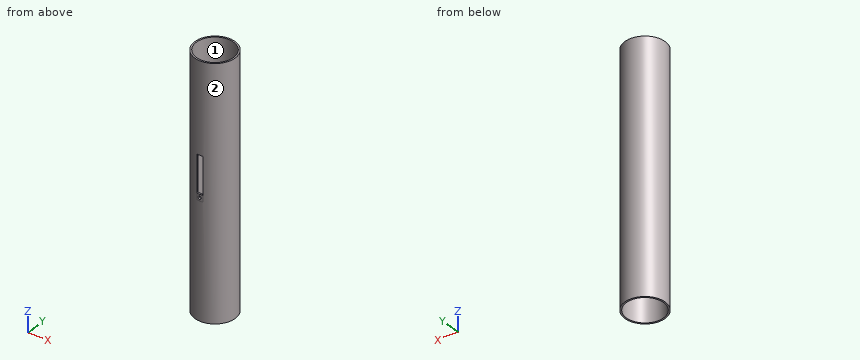
from build123d import *

# Parameters (mm, degrees)
F0_R        = 41.275
F0_R_2      = 38.1
F1_DEPTH    = 508
F3_W        = 1.5594176948
F3_H        = 13.3043527603
F4_DEPTH    = 6.35
F5_DEPTH    = 6.35
F6_R        = 3.175
F7_DEPTH    = 25.4
F8_T1_DEPTH = 52.6135854812


# Not quite as in the source:
# - a fillet or chamfer that OpenCascade refuses, or shapes differently, is made with other operations: its cross-section is extruded or revolved along the edge and cut away or added


with BuildPart() as f1:
    # F0 (on Top) → F1 (new body)
    with BuildSketch(Plane.XY):
        Circle(F0_R)
        Circle(F0_R_2, mode=Mode.SUBTRACT)
    extrude(amount=F1_DEPTH)

    # F3 (on face) → F4 (cut, symmetric)
    with BuildSketch(Plane(origin=(0, 0, 0), x_dir=(0, -1, 0), z_dir=(-1, 0, 0))):
        Polygon((63.4511685878, 247.5796341896), (63.4511685878, 323.7796341896), (25.3511685878, 323.7796341896), (25.3511685878, 247.5796341896), (39.8362353444, 247.5796341896), (41.3956530392, 247.5796341896), align=None)
        with Locations((40.6159441918, 240.9274578094)):
            Rectangle(F3_W, F3_H)
    extrude(amount=F4_DEPTH, both=True, mode=Mode.SUBTRACT)

    # F3 (on face) → F5 (join, symmetric)
    with BuildSketch(Plane(origin=(0, 0, 0), x_dir=(0, -1, 0), z_dir=(-1, 0, 0))):
        with Locations((40.6159441918, 240.9274578094)):
            Rectangle(F3_W, F3_H)
    extrude(amount=F5_DEPTH, both=True)

    # F6 (on face) → F7 (cut)
    with BuildSketch(Plane.XZ.offset(41.3956530392)):
        with Locations((0, 241.0158216953)):
            Circle(F6_R)
    extrude(amount=-F7_DEPTH, mode=Mode.SUBTRACT)

    # F8: fillet of radius 50.8 on 2 edges, made by hand

    # F8_s2 → F8_t1 (cut)
    with BuildSketch(Plane.XY.offset(214.6206650688)):
        with BuildLine():
            ThreePointArc((-6.35, -40.7836134373), (-2.4309704551, -41.2424120087), (1.5118465442, -41.3956530392))
            Line((1.5118465442, -41.3956530392), (-6.35, -41.3956530392))
            Line((-6.35, -41.3956530392), (-6.35, -40.7836134373))
        make_face()
        with BuildLine():
            ThreePointArc((6.35, -40.7836134373), (2.4309704551, -41.2424120087), (-1.5118465442, -41.3956530392))
            Line((-1.5118465442, -41.3956530392), (6.35, -41.3956530392))
            Line((6.35, -41.3956530392), (6.35, -40.7836134373))
        make_face()
    extrude(amount=F8_T1_DEPTH, mode=Mode.SUBTRACT)


solid = f1.part
Can you work these out from the model? Positions are in its coordinate system, mm. Face numbers are marked on the shaded views. Coordinates: 2 decimals unless noted, no trailing zeros. Order: outer loops, then holes, each group sorted by start corner. A loop starts at its lowest first (then second) coordinate and runs counter-clockwise, first axis right, second up. Notation, with made-up numbers: (38.5, 5.25) - (62.5, 5.25) arc R27 cw to (62.5, 40.25) - close; hole circle Ø7 at (-13.75, -24). An arc over 180 degrees is marked (long way). Answer as a JSON object with one key per item and string values. Group by question number.
Q1. Will these pins go through, and if not, where does the flat tip stop? P1, Ø10, axis at y = 12.5, z = 208.5, coming from the -X side; P2, Ø4, axis at x = 18, z = 199, coming from the -Y side; P3, Ø2.5, axis at y = -39.5, z = 270, coming from the +X side.
Q2. We'd pull the mould along X, two halves only. Please class the marked faces 1 and 2: +X half, -X half, draft (parallel to the pull), parting line (faces both ways), or undercut.
Q3. Imagine slicing it at C-C (z = 37). Please give me the cut outline in (x, y) (3 decimals), and give its area (3 significant figures).
Q4. Imagine slicing it at B-B (x = 21). Please give me the cut outline in (y, z), and give its area (3 significant figures).
Q5. I need wall thicknesses on line 1 (Y direction, x = 0, z = 182) (3 decimals); line 2 (Y direction, x = 34, z = 312); line 3 (X direction, y = 16, z = 402.5). Which ranges of each line are inside material? Lowest first, please. Write a range as from..to.
Q6. Imagine slicing it at A-A (y = 0). Please give me the cut outline in (x, z) (3 decimals).
Determined:
{
 "1": {"P1": "stops at x = -40.59", "P2": "stops at y = -38.05", "P3": "stops at x = 15.51"},
 "2": {"face 1": "undercut", "face 2": "parting line"},
 "3": {"outline": "circle Ø82.55 at (0, 0); hole circle Ø76.2 at (0, 0)", "area": "792 mm2"},
 "4": {"outline": "(-35.53, 0) - (-31.79, 0) - (-31.79, 508) - (-35.53, 508) - close; (31.79, 0) - (35.53, 0) - (35.53, 508) - (31.79, 508) - close", "area": "3,800 mm2"},
 "5": {"line 1": "y = -41.275..-38.1, 38.1..41.275", "line 2": "y = -23.4..-17.19, 17.19..23.4", "line 3": "x = -38.05..-34.58, 34.58..38.05"},
 "6": {"outline": "(-41.275, 0) - (-38.1, 0) - (-38.1, 508) - (-41.275, 508) - close; (38.1, 0) - (41.275, 0) - (41.275, 508) - (38.1, 508) - close"}
}
